CAD build for the part. Positions are in the model's coordinates, mm. Give positions to 0.01 mm unless a question says otherwise; leave off trailing zeros. Loops run counter-clockwise (first coordinate to the right, second up) from the corner with the lowest first, then second, coordinate; pieces in that order, holes last.
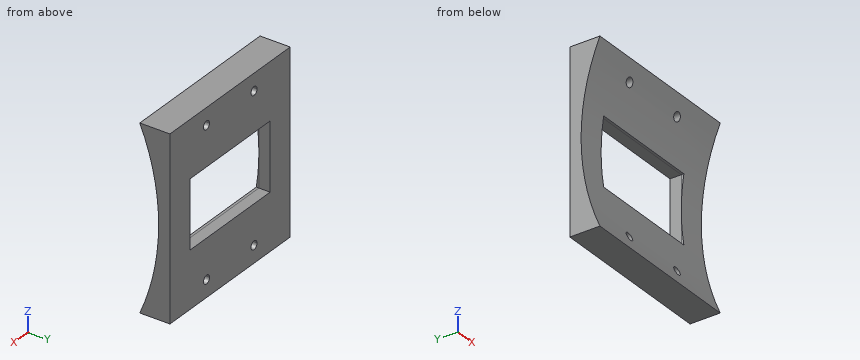
Autodesk Inventor part; units mm, degrees
ref_plane "YZ Plane" through (0, 0, 0) normal (1, 0, 0) x (0, 1, 0)
ref_plane "XZ Plane" through (0, 0, 0) normal (0, 1, 0) x (-1, 0, 0)
ref_plane "XY Plane" through (0, 0, 0) normal (0, 0, 1) x (1, 0, 0)
sketch "Sketch1" plane through (0, 0, 0) normal (0, 1, 0) x (-1, 0, 0)
  line L0 (4.7412, 12.4222) -> (-10.2588, 12.4222)
  line L1 (-10.2588, 12.4222) -> (-10.2588, -3.5778)
  line L2 (-10.2588, -3.5778) -> (4.7412, -3.5778)
  line L3 (4.7412, -3.5778) -> (4.7412, 12.4222)
  line L4 (2.2412, 7.4222) -> (-7.7588, 7.4222)
  line L5 (-7.7588, 7.4222) -> (-7.7588, 1.4222)
  line L6 (-7.7588, 1.4222) -> (2.2412, 1.4222)
  line L7 (2.2412, 1.4222) -> (2.2412, 7.4222)
  circle A0 centre (0.2287, 10.9222) radius 0.375
  circle A1 centre (-5.6963, 10.9222) radius 0.375
  circle A2 centre (0.2287, -2.0628) radius 0.375
  circle A3 centre (-5.6963, -2.0628) radius 0.375
  point P0 (0, 0)
  dimension "d0" = 15
  dimension "d1" = 16
  dimension "d2" = 10
  dimension "d3" = 6
  dimension "d4" = 2.5
  dimension "d5" = 5
  dimension "d6" = 0.75
  dimension "d7" = 4.5125
  dimension "d8" = 1.5
  dimension "d11" = 5.925
  dimension "d14" = 12.985
extrude "Extrusion1" add sketch "Sketch1" along normal blind 1
sketch "Sketch2" plane through (-4.7412, 0, -3.5778) normal (-1, 0, 0) x (0, 0, 1)
  circle A0 centre (8, -20) radius 20
  line L0 (16, 0) -> (16, 1)
  line L1 (16, 0) -> (16, -1.6697)
  line L2 (16, 0) -> (0, 0)
  line L3 (0, 0) -> (0, -1.6697)
  arc A1 (16, -1.6697) -> (0, -1.6697) centre (8, -20) ccw
  point P0 (3.5778, 0)
  point P1 (8, 0)
extrude "Extrusion2" add sketch "Sketch2" against normal up to surface (15 mm away) contours A0 L2 L1 | L3 L2 A0
sketch "Sketch3" plane through (0, 1, 0) normal (0, 1, 0) x (1, 0, 0)
  circle A0 centre (-0.2287, -10.9222) radius 0.375
  circle A1 centre (5.6963, -10.9222) radius 0.375
  circle A2 centre (-0.2287, 2.0628) radius 0.375
  circle A3 centre (5.6963, 2.0628) radius 0.375
  line L0 (-2.2412, -1.4222) -> (7.7588, -1.4222)
  line L1 (-2.2412, -7.4222) -> (-2.2412, -1.4222)
  line L2 (7.7588, -7.4222) -> (-2.2412, -7.4222)
  line L3 (7.7588, -1.4222) -> (7.7588, -7.4222)
  line L4 (-2.2412, -7.4222) -> (7.7588, -7.4222)
  line L5 (7.7588, -7.4222) -> (7.7588, -1.4222)
  line L6 (7.7588, -1.4222) -> (-2.2412, -1.4222)
  line L7 (-2.2412, -1.4222) -> (-2.2412, -7.4222)
  circle A4 centre (5.6963, 2.0628) radius 0.375
  circle A5 centre (-0.2287, 2.0628) radius 0.375
  circle A6 centre (-0.2287, -10.9222) radius 0.375
  circle A7 centre (5.6963, -10.9222) radius 0.375
  point P0 (0, 0)
extrude "Extrusion3" cut sketch "Sketch3" against normal through all
properties part number "Viewing Mirror Holder Mount"
1. Saw through at D-D, the plane y = -0.9. List the corners of the cut face in (x, z) (3 decimals).
Responses:
outline: (-4.741, -3.578) - (10.259, -3.578) - (10.259, -1.51) - (-4.741, -1.51) - close; (-4.741, 10.354) - (10.259, 10.354) - (10.259, 12.422) - (-4.741, 12.422) - close; hole circle Ø0.75 at (-0.229, -2.063); hole circle Ø0.75 at (-0.229, 10.922); hole circle Ø0.75 at (5.696, -2.063); hole circle Ø0.75 at (5.696, 10.922)
2. Probe line 1 along Z through (x, y) = (5.5, -0.1); line 2 along Y through (x, z) = (9, 4); line 3 along Z through (x, y) = (2.25, -1.5). List the from-to ranges inside material, lowest first.
Responses:
line 1: z = -3.58 to -2.38, -1.74 to 1.42, 7.42 to 10.6, 11.24 to 12.42
line 2: y = 0 to 1
line 3: z = -3.58 to -3.18, 12.02 to 12.42
3. Drop flat-ended pins along their axis: pin 1 (2 mm diameter, centred on x = 3.5, z = 9, fed in from -Y); pin 2 (1.5 mm diameter, centred on x = 6, z = 9, fed in from -Y). Give the stop position or say it passes through.
Responses:
pin 1: stops at y = -0.79
pin 2: stops at y = -0.72
4. Saw through at A-A, the plane x = -1. List the corners of the cut face in (y, z).
Responses:
outline: (-1.67, -3.58) - (1, -3.58) - (1, 1.42) - (-0.23, 1.42) arc R20 cw to start; (-1.67, 12.42) arc R20 cw to (-0.23, 7.42) - (1, 7.42) - (1, 12.42) - close
5. Saw through at C-C, the plane z = 4. List the corners of the cut face in (x, y), and give its area (3 significant figures).
Responses:
outline: (-4.74, 0) - (-2.24, 0) - (-2.24, 1) - (-4.74, 1) - close; (7.76, 0) - (10.26, 0) - (10.26, 1) - (7.76, 1) - close
area: 5.02 mm2
6. Saw through at B-B, the plane y = 0.45. List the corners of the cut face in (x, z) (3 decimals), and give its area (3 significant figures).
Responses:
outline: (-4.741, -3.578) - (10.259, -3.578) - (10.259, 12.422) - (-4.741, 12.422) - close; hole (-2.241, 1.422) - (7.759, 1.422) - (7.759, 7.422) - (-2.241, 7.422) - close; hole circle Ø0.75 at (-0.229, -2.063); hole circle Ø0.75 at (-0.229, 10.922); hole circle Ø0.75 at (5.696, -2.063); hole circle Ø0.75 at (5.696, 10.922)
area: 178 mm2
